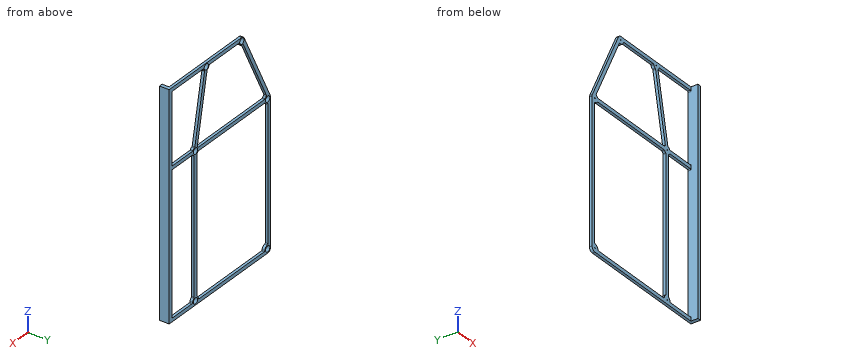
```python
from build123d import *

# Parameters (mm, degrees)
SKETCH2_R           = 0.5
BOSS_EXTRUDE1_DEPTH = 3
SKETCH3_W           = 4
SKETCH3_H           = 250.248923326
BOSS_EXTRUDE2_DEPTH = 8
CHAMFER1_SIZE       = 2.8
FILLET1_R           = 1


with BuildPart() as part:
    # Sketch2 → Boss-Extrude1 (new body)
    with BuildSketch(Plane(origin=(0, 0, 0), x_dir=(1, 0, 0), z_dir=(0, 1, 0))):
        with BuildLine():
            Line((4, -250.248923326), (4, 0))
            Line((4, 0), (0, 0))
            Line((0, 0), (-148.5, 0))
            ThreePointArc((-148.5, 0), (-151.681980515, -1.318019485), (-153, -4.5))
            Line((-153, -4.5), (-153, -164.5))
            ThreePointArc((-153, -164.5), (-152.88121444, -165.527112473), (-152.531128874, -166.5))
            Line((-152.531128874, -166.5), (-112.082261174, -248.027299256))
            ThreePointArc((-112.082261174, -248.027299256), (-110.60761765, -249.648431345), (-108.5, -250.248923326))
            Line((-108.5, -250.248923326), (4, -250.248923326))
        make_face()
        with Locations((-148.5, -4.5)):
            Circle(SKETCH2_R, mode=Mode.SUBTRACT)
        with Locations((-36.75, -4.5)):
            Circle(SKETCH2_R, mode=Mode.SUBTRACT)
        with Locations((-36.75, -164.5)):
            Circle(SKETCH2_R, mode=Mode.SUBTRACT)
        with Locations((-148.5, -164.5)):
            Circle(SKETCH2_R, mode=Mode.SUBTRACT)
        with Locations((-108.5, -246.25)):
            Circle(SKETCH2_R, mode=Mode.SUBTRACT)
        with Locations((-53.5, -246.25)):
            Circle(SKETCH2_R, mode=Mode.SUBTRACT)
        with BuildLine():
            Line((0, -4), (0, -162.5))
            Line((0, -162.5), (-32.718871126, -162.5))
            ThreePointArc((-32.718871126, -162.5), (-33.568019485, -161.318019485), (-34.75, -160.468871126))
            Line((-34.75, -160.468871126), (-34.75, -8.531128874))
            ThreePointArc((-34.75, -8.531128874), (-32.799693914, -6.655245189), (-32.277864045, -4))
            Line((-32.277864045, -4), (0, -4))
        make_face(mode=Mode.SUBTRACT)
        with BuildLine():
            Line((-144.027864045, -4), (-41.222135955, -4))
            ThreePointArc((-41.222135955, -4), (-40.700306086, -6.655245189), (-38.75, -8.531128874))
            Line((-38.75, -8.531128874), (-38.75, -160.468871126))
            ThreePointArc((-38.75, -160.468871126), (-39.931980515, -161.318019485), (-40.781128874, -162.5))
            Line((-40.781128874, -162.5), (-144.468871126, -162.5))
            ThreePointArc((-144.468871126, -162.5), (-146.344754811, -160.549693914), (-149, -160.027864045))
            Line((-149, -160.027864045), (-149, -8.972135955))
            ThreePointArc((-149, -8.972135955), (-145.318019485, -7.681980515), (-144.027864045, -4))
        make_face(mode=Mode.SUBTRACT)
        with BuildLine():
            Line((-32.718871126, -166.5), (0, -166.5))
            Line((0, -166.5), (0, -246.248923326))
            Line((0, -246.248923326), (-49.501076819, -246.248923326))
            ThreePointArc((-49.501076819, -246.248923326), (-49.852891921, -244.609880972), (-50.845628636, -243.25906362))
            Line((-50.845628636, -243.25906362), (-35.599844174, -168.850533482))
            ThreePointArc((-35.599844174, -168.850533482), (-33.905236442, -167.986734905), (-32.718871126, -166.5))
        make_face(mode=Mode.SUBTRACT)
        with BuildLine():
            Line((-146.960287228, -168.728390306), (-110.2763347, -242.667260434))
            ThreePointArc((-110.2763347, -242.667260434), (-106.39238235, -242.851568655), (-104.501076819, -246.248923326))
            Line((-104.501076819, -246.248923326), (-57.498923181, -246.248923326))
            ThreePointArc((-57.498923181, -246.248923326), (-56.743672678, -243.911202162), (-54.764220792, -242.456171649))
            Line((-54.764220792, -242.456171649), (-39.518436329, -168.047641511))
            ThreePointArc((-39.518436329, -168.047641511), (-40.236734905, -167.344763558), (-40.781128874, -166.5))
            Line((-40.781128874, -166.5), (-144.468871126, -166.5))
            ThreePointArc((-144.468871126, -166.5), (-145.5, -167.854101966), (-146.960287228, -168.728390306))
        make_face(mode=Mode.SUBTRACT)
    extrude(amount=BOSS_EXTRUDE1_DEPTH)

    # Sketch3 → Boss-Extrude2 (add)
    with BuildSketch(Plane.XZ):
        with Locations((2, 125.124461663)):
            Rectangle(SKETCH3_W, SKETCH3_H)
    extrude(amount=BOSS_EXTRUDE2_DEPTH)

    # Chamfer1
    chamfer1_edges = [part.edges().sort_by_distance(p)[0] for p in [
        (-109, 3, 246.25),
        (-54, 3, 246.25),
        (-149, 3, 4.5),
        (-37.25, 3, 4.5),
        (-37.25, 3, 164.5),
        (-149, 3, 164.5),
    ]]
    chamfer(chamfer1_edges, length=CHAMFER1_SIZE)

    # Fillet1
    fillet1_edges = [part.edges().sort_by_distance(p)[0] for p in [
        (-32.718871126, 1.5, 166.5),
        (-35.599844174, 1.5, 168.850533482),
        (-50.845628636, 1.5, 243.25906362),
        (-49.501076819, 1.5, 246.248923326),
        (0, 1.5, 246.248923326),
        (0, 1.5, 166.5),
        (-32.277864045, 1.5, 4),
        (-34.75, 1.5, 8.531128874),
        (-34.75, 1.5, 160.468871126),
        (-32.718871126, 1.5, 162.5),
        (0, 1.5, 162.5),
        (0, 1.5, 4),
        (-144.027864045, 1.5, 4),
        (-149, 1.5, 8.972135955),
        (-149, 1.5, 160.027864045),
        (-144.468871126, 1.5, 162.5),
        (-40.781128874, 1.5, 162.5),
        (-38.75, 1.5, 160.468871126),
        (-38.75, 1.5, 8.531128874),
        (-41.222135955, 1.5, 4),
        (-57.498923181, 1.5, 246.248923326),
        (-54.764220792, 1.5, 242.456171649),
        (-39.518436329, 1.5, 168.047641511),
        (-40.781128874, 1.5, 166.5),
        (-144.468871126, 1.5, 166.5),
        (-146.960287228, 1.5, 168.728390306),
        (-110.2763347, 1.5, 242.667260434),
        (-104.501076819, 1.5, 246.248923326),
    ]]
    fillet(fillet1_edges, radius=FILLET1_R)


solid = part.part
```
Build history of the part. All positions in model axes, mm. Give positions to 0.01 mm unless a question says otherwise; leave off trailing zeros. Order: outer loops, then holes, each group sorted by start corner. A loop starts at its lowest first (then second) coordinate and runs counter-clockwise, first axis right, second up. Notation, with made-up numbers: M -32,-8.75 L 25,-8.75 A16 ccw 25,7.25 Z; hole C 1,51 d3. An arc over 180 degrees is marked long. Return JSON: item names as keys, results as strings.
Q1. Band-saw the part on A-A (z = 150). Give the cut face in (x, y).
Answer list:
{"outline": "M -153,0 L -149,0 L -149,3 L -153,3 Z; M -38.75,0 L -34.75,0 L -34.75,3 L -38.75,3 Z; M 0,-8 L 4,-8 L 4,3 L 0,3 Z"}
Q2. Wall check: probe 1 along X at (y, z) = (0.75, 65); probe 2 along X at (y, z) = (0.1, 164.5); probe 3 along Z at (x, y) = (-18, 2.5). Give the ranges that are in metal, low to high. Write a range as from..to.
Answer list:
{"probe 1": "x = -153..-149, -38.75..-34.75, 0..4", "probe 2": "x = -153..-149, -148..-37.25, -36.25..4", "probe 3": "z = 0..4, 162.5..166.5, 246.25..250.25"}
Q3. Band-saw the part on C-C (y = -4). Give the cut face in (x, z).
Answer list:
{"outline": "M 0,0 L 4,0 L 4,250.25 L 0,250.25 Z"}
Q4. Flat gauge pins, fed straight in: pin 1 (1.5 mm diameter, centred on y = -3, z = 201.5, fed in from -X); pin 2 (4 mm diameter, centred on x = -137, y = -2.5, fed in from -Z). Where does each tip first touch, or does it go through?
Answer list:
{"pin 1": "stops at x = 0", "pin 2": "passes through"}
Q5. Band-saw the part on B-B (x = -85). Give the cut face in (y, z), then the cut area to 3 significant figures.
Answer list:
{"outline": "M 0,0 L 3,0 L 3,4 L 0,4 Z; M 0,162.5 L 3,162.5 L 3,166.5 L 0,166.5 Z; M 0,246.25 L 3,246.25 L 3,250.25 L 0,250.25 Z", "area": "36.0 mm^2"}
